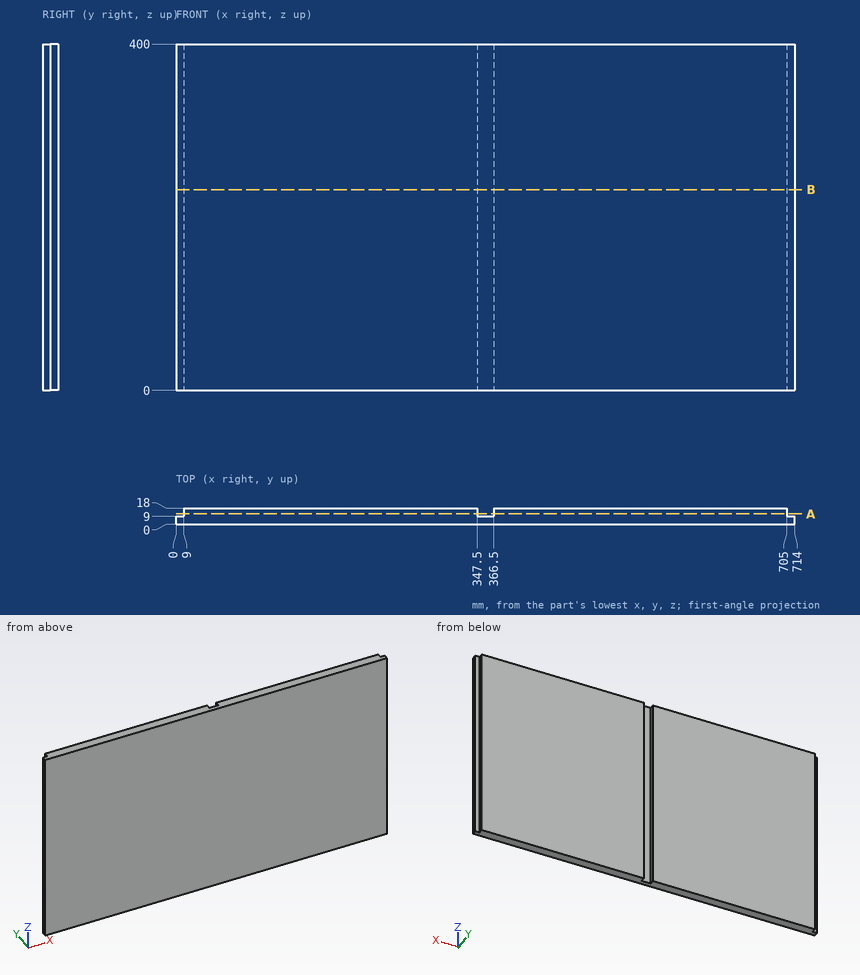
Check sheet for the drawn part. Datum: minimum x, y, z corner. Units: mm. Round coordinates to 2 decimals unless told otherwise and drop trailing zeros. Loops run counter-clockwise (first coordinate to the right, second up) from the corner with the lowest first, then second, coordinate; pieces in that order, holes last. Notation, with made-up numbers: M 31,46.25 L 86,46.25 A13 cw 86,54.25 Z; hole C 2,31.25 d9. An arc over 180 degrees is marked long. Write each question's results on one line, items separated by ' | '.
1) Section check A-A on y = 11.75. Record the boundary of the cut face in (x, z), then the cut area to 3 significant figures.
Checks:
outline: M 9,0 L 347.5,0 L 347.5,400 L 9,400 Z; M 366.5,0 L 705,0 L 705,400 L 366.5,400 Z | area: 271,000 mm2
2) Section check B-B on z = 232. Record the boundary of the cut face in (x, y).
Checks:
outline: M 0,0 L 714,0 L 714,9 L 705,9 L 705,18 L 366.5,18 L 366.5,9 L 347.5,9 L 347.5,18 L 9,18 L 9,9 L 0,9 Z
3) Gauge pin test, flat ends, axial feed: P1, Ø4.5, axis at y = 15.5, z = 211.5, coming from the -X side; P2, Ø7, axis at x = 3.5, z = 107, coming from the +Y side; P3, Ø4.5, axis at y = 12, z = 284, coming from the +X side. Record the tip position at first contact, or that the pin passes through.
Checks:
P1: stops at x = 9 | P2: stops at y = 9 | P3: stops at x = 705
4) Scan line: L1, parallel to X at y = 12, z = 165. Record every from-to range of solid material in increasing order. Write a range as from..to.
Checks:
L1: x = 9..347.5, 366.5..705
